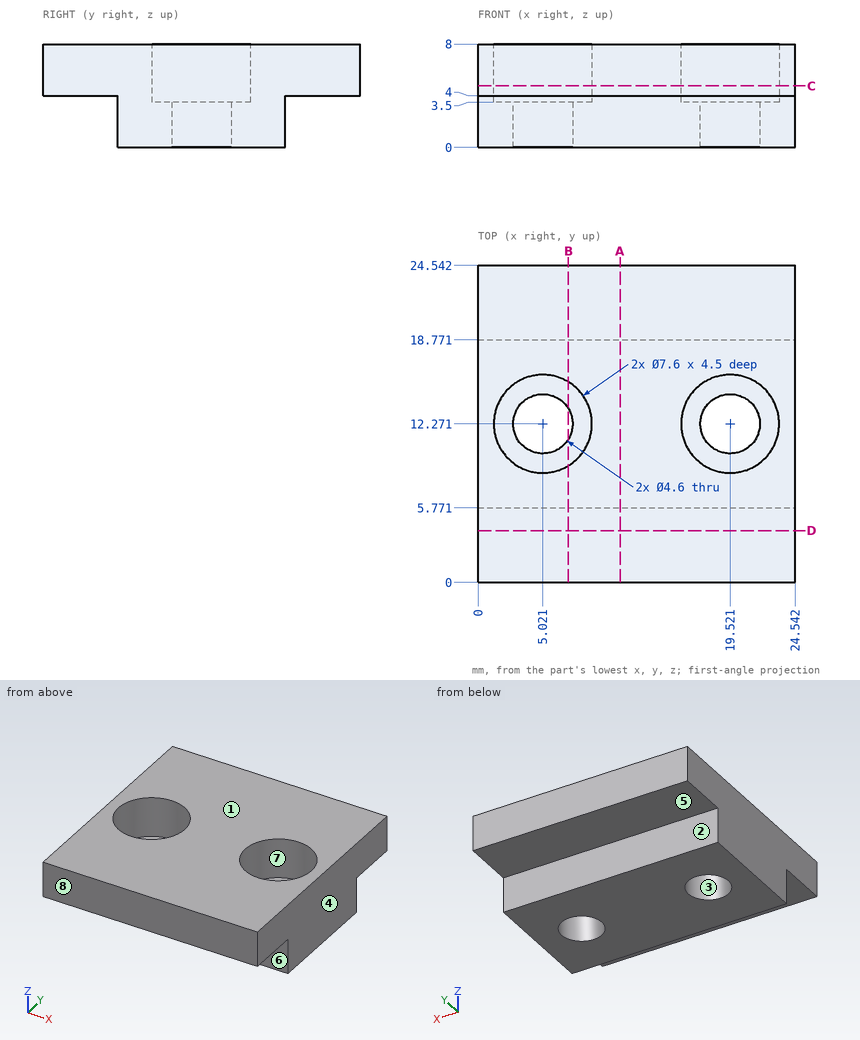
Study the drawing (mm; zero at the part's minimum x, y, z) and answer. A direction names the side the tool comes from. Give positions to 0.01 mm unless a question says otherwise; leave off trailing zeros. Write each loop counter-clockwise with the first axis right and the second up, starting at its lowest first coordinate (ties: lowest second). Pieces come first, ordered by that corner, then holes. Notation, with made-up numbers: (-19, 61.5) - (-13, 61.5) arc R12 ccw to (-13, 67.5) - close; hole circle Ø9 at (-30.75, 5). An arc over 180 degrees is marked (long way). Use a Markdown table: item, result.
1. For a pull along Y with two mould halves and no side action, classify the marked faces 1, 2 and 3 as released by +Y, released by -Y, zero draft, split by the parting line, or undercut.
Values follow:
| item | result |
|---|---|
| face 1 | zero draft |
| face 2 | released by +Y |
| face 3 | undercut |
2. Section B-B on x = 7 is taken. Write down the section's boundary in (y, z) (3 decimals).
Values follow:
| item | result |
|---|---|
| outline | (0, 4) - (5.771, 4) - (5.771, 0) - (11.099, 0) - (11.099, 3.5) - (9.027, 3.5) - (9.027, 8) - (0, 8) - close; (13.443, 0) - (18.771, 0) - (18.771, 4) - (24.542, 4) - (24.542, 8) - (15.515, 8) - (15.515, 3.5) - (13.443, 3.5) - close |
3. A tool of negligible diameter and unlimited length cuts with its end or side. For the marked faces 4, 5, 6, 7 and 8, from which of +Z, -Z, +X, -X, +Y, -Y can it reach the whole face along a straight path? Write none if from no direction.
Values follow:
| item | result |
|---|---|
| face 4 | +Z, -Z, +X, +Y, -Y |
| face 5 | -Z, +X, -X, +Y |
| face 6 | -Z, +X, -X, -Y |
| face 7 | +Z |
| face 8 | +Z, -Z, +X, -X, -Y |
4. Find the intervals of material crossed by probe 1 along X at (y, z) = (10.5, 3); probe 2 along Y at (x, z) = (2, 7.75); probe 3 along Z at (x, y) = (19.25, 3), in increasing order. Write a range as from..to.
Values follow:
| item | result |
|---|---|
| probe 1 | x = 0..3.55, 6.49..18.05, 20.99..24.54 |
| probe 2 | y = 0..9.97, 14.58..24.54 |
| probe 3 | z = 4..8 |
5. Section D-D on y = 4 is taken. Write down the section's boundary in (x, z).
Values follow:
| item | result |
|---|---|
| outline | (0, 4) - (24.54, 4) - (24.54, 8) - (0, 8) - close |
6. Section C-C on z = 4.75 is taken. Write down the section's boundary in (x, y).
Values follow:
| item | result |
|---|---|
| outline | (0, 0) - (24.54, 0) - (24.54, 24.54) - (0, 24.54) - close; hole circle Ø7.6 at (5.02, 12.27); hole circle Ø7.6 at (19.52, 12.27) |
7. Section A-A on x = 11 is taken. Write down the section's boundary in (y, z), plus the area to 3 significant figures.
Values follow:
| item | result |
|---|---|
| outline | (0, 4) - (5.77, 4) - (5.77, 0) - (18.77, 0) - (18.77, 4) - (24.54, 4) - (24.54, 8) - (0, 8) - close |
| area | 150 mm² |
8. Each of these flat-tipped pins is pushed along its axis until it touches: P1, Ø3, axis at x = 16.5, z = 2, coming from the +Y side; P2, Ø2.5, axis at x = 7, y = 11.5, coming from the +Z side; P3, Ø4.5, axis at x = 16.5, y = 22.5, coming from the -Z side. Where does it stop, or does it pass through?
Values follow:
| item | result |
|---|---|
| P1 | stops at y = 18.77 |
| P2 | stops at z = 3.5 |
| P3 | stops at z = 4 |
